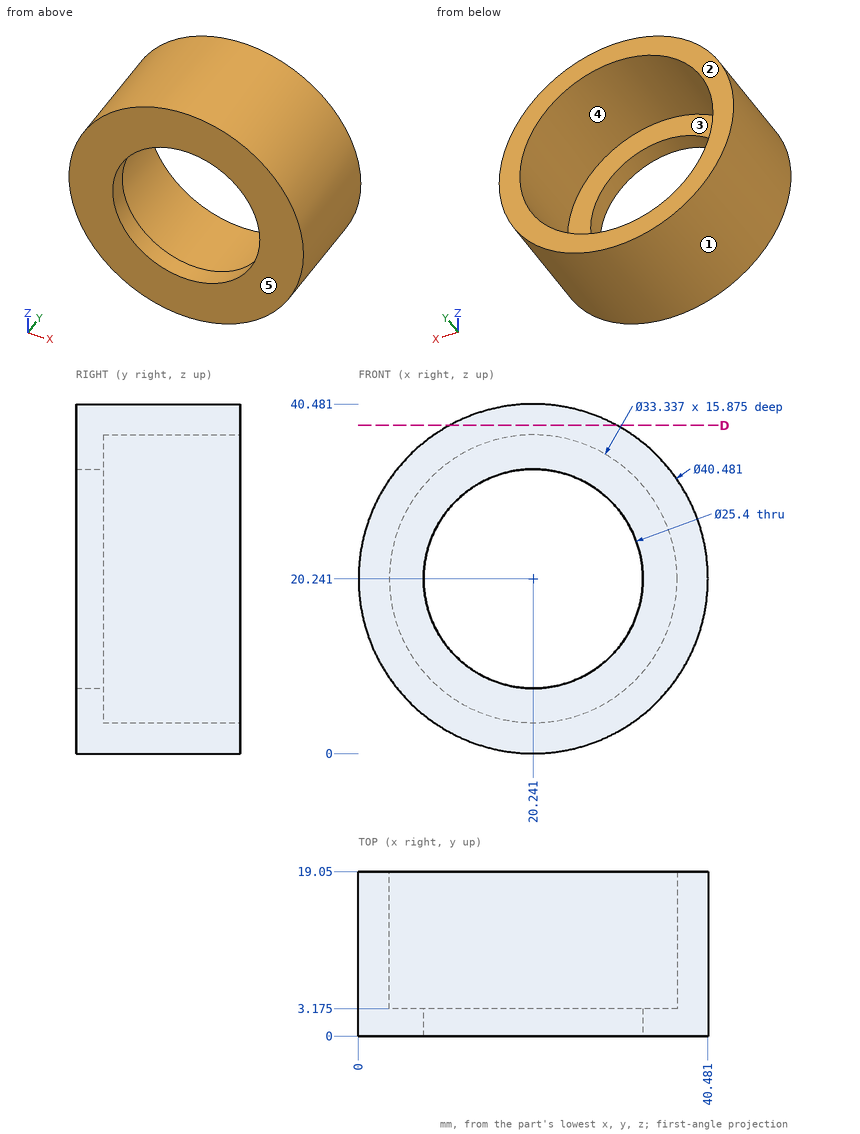
Study the drawing (mm; zero at the part's minimum x, y, z) and answer. A direction names the side the tool comes from. Give positions to 0.01 mm unless a question says otherwise; leave off trailing zeros. Order: outer loops, then holes, each group sorted by start corner. A loop starts at its lowest first (then second) coordinate and runs counter-clockwise, first axis right, second up. Notation, with made-up numbers: (40.25, 80) - (73.25, 80) arc R12 ccw to (73.25, 101) - close; hole circle Ø7 at (88.25, 5.5). An arc over 180 degrees is marked (long way). Answer in a Markdown table with one row per item. Add a question column.
Q1. Which of the six approach directions +Z, -Z, +X, -X, +Y, -Y give full straight-line access (tool end or side, diameter ignored) to the marked faces 4 and 5?
Q2. For a pull along X with two mould halves and no side action, classify the marked faces 1, 2 and 3 as released by +X, released by -X, zero draft, split by the parting line, or undercut.
Q3. Given P1, Ø4, axis at y = 3.5, z = 23, coming from the -X side; P2, Ø8, axis at x = 13, y = 13, coming from the -Z side; P3, Ø1.5, axis at x = 11, y = 11, coming from the -Z side, each flat-ended and moving along its own axis, determine where each tip first touches the part or whether it passes through.
Q4. Find the intervals of material crossed by line 1 along Y through (x, z) = (24, 36) (1 decimal); line 2 along Z through (x, y) = (29, 11.75) (1 decimal); line 3 along X through (y, z) = (8.5, 5) (1 decimal), in increasing order. Write a range as [from, to].
Q5. The part is cut by section D-D (z = 38). Determine the outline of the cut face in (x, y), then the cut area to 3 significant figures.
Determined:
| question | item | result |
|---|---|---|
| 1 | face 4 | +Y |
| 1 | face 5 | +Z, -Z, +X, -X, -Y |
| 2 | face 1 | split by the parting line |
| 2 | face 2 | zero draft |
| 2 | face 3 | undercut |
| 3 | P1 | stops at x = 0.01 |
| 3 | P2 | stops at z = 0.26 |
| 3 | P3 | stops at z = 1.87 |
| 4 | line 1 | y = [0, 3.2] |
| 4 | line 2 | z = [2, 6.1], [34.4, 38.5] |
| 4 | line 3 | x = [6.9, 13.5], [27, 33.6] |
| 5 | outline | (10.53, 0) - (29.95, 0) - (29.95, 19.05) - (10.53, 19.05) - close |
| 5 | area | 370 mm² |
